Check sheet for the modelled part. Datum: model origin and axes. Units: mm. A direction names the side the tool comes from. Round coordinates to 2 decimals unless told otherwise and drop trailing zeros. Write each loop counter-clockwise with the first axis right and the second up, starting at its lowest first coordinate (ties: lowest second). Pieces come first, ordered by that corner, then holes. Notation, with made-up numbers: (3.25, 51) -> (19.25, 51) arc R8 cw to (19.25, 57) -> close; hole circle Ø6 at (-13.5, 47.5). An arc over 180 degrees is marked (long way). Write item = value, one per line.
from build123d import *

# Parameters (mm, degrees)
CHAMFER_1_SIZE         = 0.3
CUT_EXTRUDE_2_DEPTH    = 1
HOLE_WIZARD_M3_1_D     = 2.5
HOLE_WIZARD_M3_1_DEPTH = 8.5
HOLE_WIZARD_M3_1_TIP   = 0.751075774


with BuildPart() as part:
    # ｽｹｯﾁ1 → 回転1 (revolve)
    with BuildSketch(Plane.XY):
        Polygon((0, -5), (-1.5, -5), (-1.5, 0), (-3, 0), (-3, 11), (0, 11), align=None)
    revolve(axis=Axis((0, 16.004822162, 0), (0, -1, 0)))

    # 面取り1
    chamfer_1_edges = [part.edges().sort_by_distance(p)[0] for p in [
        (3, 11, 0),
        (3, 0, 0),
        (1.5, -5, 0),
    ]]
    chamfer(chamfer_1_edges, length=CHAMFER_1_SIZE)

    # ｽｹｯﾁ2 → ｶｯﾄ - 押し出し2 (cut)
    with BuildSketch(Plane(origin=(0, 11, 0), x_dir=(1, 0, 0), z_dir=(0, 1, 0))):
        with BuildLine():
            Line((0.5, -2.958039892), (0.5, 2.958039892))
            ThreePointArc((0.5, 2.958039892), (0, 3), (-0.5, 2.958039892))
            Line((-0.5, 2.958039892), (-0.5, -2.958039892))
            ThreePointArc((-0.5, -2.958039892), (0, -3), (0.5, -2.958039892))
        make_face()
    extrude(amount=-CUT_EXTRUDE_2_DEPTH, mode=Mode.SUBTRACT)

    # M3 ねじ穴1
    with Locations(Plane(origin=(0, 11, 0), x_dir=(1, 0, 0), z_dir=(0, 1, 0))):
        with Locations((0, 0)):
            Hole(HOLE_WIZARD_M3_1_D / 2, depth=HOLE_WIZARD_M3_1_DEPTH)
            with Locations((0, 0, -(HOLE_WIZARD_M3_1_DEPTH + HOLE_WIZARD_M3_1_TIP / 2))):  # 118° drill point
                Cone(0, HOLE_WIZARD_M3_1_D / 2, HOLE_WIZARD_M3_1_TIP, mode=Mode.SUBTRACT)


solid = part.part
(1) Release check for a two-part mould opening along X. For faces 4 (the flat face through (0, -5, 0)), 5 (the cylindrical face through (-1.19, 6.69, -0.38)), 6 (the conical face through (-2.81, 10.89, 0.06)) record: pulls with the +X half, pulls with the -X half, needs draft (parallel to the pull), parting line crosses it, or undercut.
Worked answers:
face_4 = needs draft
face_5 = undercut
face_6 = pulls with the -X half
(2) Sectioned sample at A-A on y = 3. Enter the section's corners in (x, z).
Worked answers:
outline = circle Ø6 at (0, 0); hole circle Ø2.5 at (0, 0)
(3) Material ranges on L1, parallel to Z at x = 0, y = 4.5; L2, parallel to Y at x = -2.2, z = 1.25; L3, parallel to X at y = 8.25, z = 2.75, recorded low to high. Write a range as [from, to].
Worked answers:
L1 = [-3, -1.25], [1.25, 3]
L2 = [0, 11]
L3 = [-1.2, 1.2]
(4) Go/stop test with flat-tipped pins: P1, Ø1.1, axis at y = 10.5, z = 2, coming from the +X side; P2, Ø0.5, axis at y = 10.5, z = 2, coming from the -X side; P3, Ø0.8, axis at x = 0, z = 2, coming from the +Y side. Record where each tip stops, or that it passes through.
Worked answers:
P1 = 2.63
P2 = -2.44
P3 = 10
(5) Sectioned sample at B-B on y = -1.25. Enter the section's corners in (x, z).
Worked answers:
outline = circle Ø3 at (0, 0)
(6) Access from +Z, -Z, +X, -X, +Y, -Y to the whole of each face (thin tool, end or side, straight path). Record for faces 1 (the flat face through (-0.5, 10.5, 2)), 2 (the flat face through (2, 11, 0)), 3 (the flat face through (1.2, 0, 1.2)).
Worked answers:
face_1 = +Z, -Z, +Y
face_2 = +Z, -Z, +X, -X, +Y
face_3 = -Y
